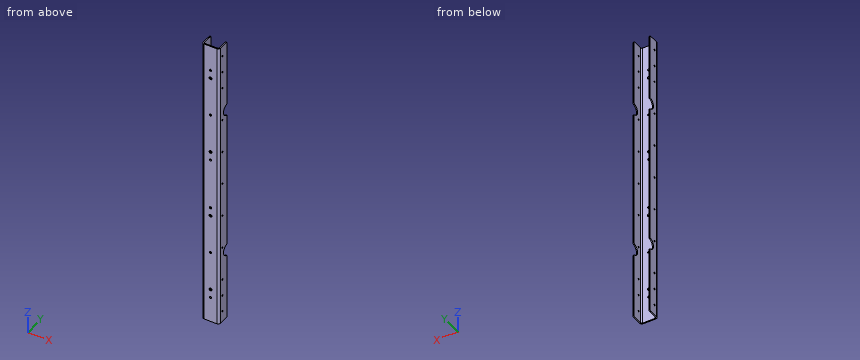
```python
from build123d import *

# Parameters (mm, degrees)
BASE_FLANGE1_DEPTH = 876.3
SKETCH6_R          = 2.4257
SKETCH6_R_2        = 17.4625
CUT_EXTRUDE1_DEPTH = 879.597712267
FILLET1_R          = 3.175
SKETCH8_R          = 3.3782
SKETCH8_R_2        = 4.3688
CUT_EXTRUDE2_DEPTH = 879.597712267


# Sheet-metal steps are written as plain solids
with BuildPart() as part:
    # Sketch1 → Base-Flange1 (new body)
    with BuildSketch(Plane.XY):
        with BuildLine():
            Line((50.8, 38.1), (50.8, 6.35))
            ThreePointArc((50.8, 6.35), (48.940128061, 1.859871939), (44.45, 0))
            Line((44.45, 0), (6.35, 0))
            ThreePointArc((6.35, 0), (1.859871939, 1.859871939), (0, 6.35))
            Line((0, 6.35), (0, 38.1))
            Line((0, 38.1), (3.175, 38.1))
            Line((3.175, 38.1), (3.175, 6.35))
            ThreePointArc((3.175, 6.35), (4.10493597, 4.10493597), (6.35, 3.175))
            Line((6.35, 3.175), (44.45, 3.175))
            ThreePointArc((44.45, 3.175), (46.69506403, 4.10493597), (47.625, 6.35))
            Line((47.625, 6.35), (47.625, 38.1))
            Line((47.625, 38.1), (50.8, 38.1))
        make_face()
    extrude(amount=BASE_FLANGE1_DEPTH)

    # Sketch6 → Cut-Extrude1 (cut, through all)
    with BuildSketch(Plane(origin=(50.8, 0, 0), x_dir=(0, 0, -1), z_dir=(1, 0, 0))):
        with Locations((-438.15, 15.875)):
            Circle(SKETCH6_R)
        with Locations((-336.55, 15.875)):
            Circle(SKETCH6_R)
        with Locations((-234.95, 15.875)):
            Circle(SKETCH6_R)
        with Locations((-133.35, 15.875)):
            Circle(SKETCH6_R)
        with Locations((-31.75, 15.875)):
            Circle(SKETCH6_R)
        with Locations((-844.55, 15.875)):
            Circle(SKETCH6_R)
        with Locations((-742.95, 15.875)):
            Circle(SKETCH6_R)
        with Locations((-641.35, 15.875)):
            Circle(SKETCH6_R)
        with Locations((-539.75, 15.875)):
            Circle(SKETCH6_R)
        with Locations((-661.3398, 38.9255)):
            Circle(SKETCH6_R_2)
        with Locations((-214.9602, 38.9255)):
            Circle(SKETCH6_R_2)
        with Locations((-793.75, 15.875)):
            Circle(SKETCH6_R)
        with Locations((-82.55, 15.875)):
            Circle(SKETCH6_R)
    extrude(amount=-CUT_EXTRUDE1_DEPTH, mode=Mode.SUBTRACT)

    # Fillet1
    fillet1_edges = [part.edges().sort_by_distance(p)[0] for p in [
        (1.5875, 38.1, 0),
        (1.5875, 38.1, 678.782777269),
        (1.5875, 38.1, 643.896822731),
        (49.2125, 38.1, 678.782777269),
        (49.2125, 38.1, 643.896822731),
        (1.5875, 38.1, 232.403177269),
        (1.5875, 38.1, 197.517222731),
        (49.2125, 38.1, 232.403177269),
        (49.2125, 38.1, 197.517222731),
        (49.2125, 38.1, 0),
        (1.5875, 38.1, 876.3),
        (49.2125, 38.1, 876.3),
    ]]
    fillet(fillet1_edges, radius=FILLET1_R)

    # Sketch8 → Cut-Extrude2 (cut, through all)
    with BuildSketch(Plane.XZ):
        with Locations(Location((25.4, 800.1, 0), (0, 0, 270))):
            Circle(SKETCH8_R)
        with Locations(Location((25.4, 774.7, 0), (0, 0, 270))):
            Circle(SKETCH8_R_2)
        with Locations(Location((25.4, 657.225, 0), (0, 0, 270))):
            Circle(SKETCH8_R)
        with Locations(Location((25.4, 514.35, 0), (0, 0, 270))):
            Circle(SKETCH8_R)
        with Locations(Location((25.4, 539.75, 0), (0, 0, 270))):
            Circle(SKETCH8_R_2)
        with Locations(Location((25.4, 336.55, 0), (0, 0, 270))):
            Circle(SKETCH8_R_2)
        with Locations(Location((25.4, 361.95, 0), (0, 0, 270))):
            Circle(SKETCH8_R)
        with Locations(Location((25.4, 219.075, 0), (0, 0, 270))):
            Circle(SKETCH8_R)
        with Locations(Location((25.4, 101.6, 0), (0, 0, 270))):
            Circle(SKETCH8_R_2)
        with Locations(Location((25.4, 76.2, 0), (0, 0, 270))):
            Circle(SKETCH8_R)
    extrude(amount=-CUT_EXTRUDE2_DEPTH, mode=Mode.SUBTRACT)


solid = part.part
```
Design review of the part built by this model. Coordinates are the model's own, in mm. Round coordinates to 2 decimals unless told otherwise and drop trailing zeros. Write each loop counter-clockwise with the first axis right and the second up, starting at its lowest first coordinate (ties: lowest second). Pieces come first, ordered by that corner, then holes. Notation, with made-up numbers: (67.25, -37) -> (79.25, -37) arc R20 cw to (79.25, -17) -> close; hole circle Ø9 at (-32, 61.25). An arc over 180 degrees is marked (long way). Write item = value, one per line. Start each with the question number.
1) Clearance check with a flat-ended pin moving along its axis: pin 1 (6 mm diameter, centred on x = 21.5, z = 666, fed in from +Y) (3 decimals). State where the tip first meets the part, or that it passes through.
2) Take a section at B-B, the plane x = 37. State the section outline as (y, z) points (3 decimals).
3) Wall thickness on probe 1 along X at (y, z) = (26, 189) (3 decimals); probe 2 along Y at (x, z) = (1.9, 844.55); probe 3 along Y at (x, z) = (24, 374) (3 decimals): over which ranges is each line inside the solid? List them lowest first. Write a range as from..to.
4) Take a section at A-A, the plane z = 598. State the section outline as (x, y) points (3 decimals).
Results list:
q1.pin_1 = 3.175
q2.outline = (0, 0) -> (3.175, 0) -> (3.175, 876.3) -> (0, 876.3) -> close
q3.probe_1 = 0..3.175, 47.625..50.8
q3.probe_2 = 1.82..13.45, 18.3..38.1
q3.probe_3 = 0..3.175
q4.outline = (0, 6.35) arc R6.35 ccw to (6.35, 0) -> (44.45, 0) arc R6.35 ccw to (50.8, 6.35) -> (50.8, 38.1) -> (47.625, 38.1) -> (47.625, 6.35) arc R3.175 cw to (44.45, 3.175) -> (6.35, 3.175) arc R3.175 cw to (3.175, 6.35) -> (3.175, 38.1) -> (0, 38.1) -> close
